Model file for the job. Use its own axes, mm. A direction names the side the tool comes from. Round coordinates to 2 decimals unless told otherwise and drop trailing zeros. Loops run counter-clockwise (first coordinate to the right, second up) from the corner with the lowest first, then second, coordinate; pieces in that order, holes last. Notation, with made-up numbers: (-30, 66) - (-4, 66) arc R28 ccw to (-4, 87) - close; hole circle Ø7 at (-14, 70). An arc over 180 degrees is marked (long way). Use one line per item in the form item = value.
from build123d import *

# Parameters (mm, degrees)
PAD001_DEPTH = 10
SKETCH002_R  = 1.7
HOLE_DEPTH   = 25
SKETCH003_R  = 2.35
POCKET_DEPTH = 5
FILLET_R     = 1


with BuildPart() as part:
    # Sketch001 → Pad001 (new body)
    with BuildSketch(Plane.XY):
        Polygon((-10, 0), (-10, -3), (-2, -3), (-2, -16), (2, -16), (2, 0), align=None)
    extrude(amount=-PAD001_DEPTH)

    # Sketch002 (on Face2 of Pad001) → Hole (cut)
    with BuildSketch(Plane.XZ.offset(3)):
        with Locations((-6, -5)):
            Circle(SKETCH002_R)
    extrude(amount=-HOLE_DEPTH, mode=Mode.SUBTRACT)

    # Sketch003 (on Face6 of Hole) → Pocket (cut)
    with BuildSketch(Plane.YZ.offset(2)):
        with Locations((-8, -5)):
            Circle(SKETCH003_R)
    extrude(amount=-POCKET_DEPTH, mode=Mode.SUBTRACT)

    # Fillet
    fillet_edges = [part.edges().sort_by_distance(p)[0] for p in [
        (0, -16, 0),
        (0, -16, -10),
    ]]
    fillet(fillet_edges, radius=FILLET_R)


solid = part.part
1. Cut at A-A, the plane y = -8. Give the cut face in (x, z), plus the area to 3 significant figures.
Geometry check:
outline = (-2, -10) - (2, -10) - (2, -7.35) - (-2, -7.35) - close; (-2, -2.65) - (2, -2.65) - (2, 0) - (-2, 0) - close
area = 21.2 mm^2
2. Cut at B-B, the plane z = -5. Give the cut face in (x, y), plus the area to 3 significant figures.
Geometry check:
outline = (-10, -3) - (-7.7, -3) - (-7.7, 0) - (-10, 0) - close; (-4.3, -3) - (-2, -3) - (-2, -5.65) - (2, -5.65) - (2, 0) - (-4.3, 0) - close; (-2, -16) - (2, -16) - (2, -10.35) - (-2, -10.35) - close
area = 59.0 mm^2
3. Pull direction X, two halves, no side cores. Call faces 3 (the cylindrical face through (-6.37, -1.52, -6.66)), 4 (the cylindrical face through (0.028, -10.348, -4.897)), 5 (the flat face through (2, -10, -3)): +X half, -X half, draft (parallel to the pull), parting line (faces both ways), or undercut.
Geometry check:
face_3 = undercut
face_4 = draft
face_5 = +X half
4. Flat gauge pins, fed straight in: pin 1 (5 mm diameter, centred on y = -3.5, z = -5, fed in from -X); pin 2 (2.5 mm diameter, centred on x = -6, z = -5, fed in from +Y); pin 3 (6 mm diameter, centred on y = -9, z = -4, fed in from -X). Where does each tip first touch, or does it go through?
Geometry check:
pin_1 = -10
pin_2 = through
pin_3 = -2
5. Tool access for faces 1 (the flat face through (0, -16, -5)), 2 (the flat face through (-8, -3, -5)): list every direction of +Z, -Z, +X, -X, +Y, -Y with a clear straight run to the whole face (end or side of a thin tool).
Geometry check:
face_1 = +Z, -Z, +X, -X, -Y
face_2 = +Z, -Z, -X, -Y
6. Cut at C-C, the plane x = -6. Give the cut face in (y, z), plus the area to 3 significant figures.
Geometry check:
outline = (-3, -10) - (0, -10) - (0, -6.7) - (-3, -6.7) - close; (-3, -3.3) - (0, -3.3) - (0, 0) - (-3, 0) - close
area = 19.8 mm^2
7. Wall check: probe 1 along Z at (x, y) = (-6, -0.8); probe 2 along X at (y, z) = (-5.25, -8.5); probe 3 along Z at (x, y) = (0.55, -8). Give the ranges that are in metal, low to high.
Geometry check:
probe_1 = -10 to -6.7, -3.3 to 0
probe_2 = -2 to 2
probe_3 = -10 to -7.35, -2.65 to 0
8. Cut at D-D, the plane y = -1.5. Give the cut face in (x, z).
Geometry check:
outline = (-10, -10) - (2, -10) - (2, 0) - (-10, 0) - close; hole circle Ø3.4 at (-6, -5)
